Build history of the part. All positions in model axes, mm. Face numbers are marked on the shaded views. A direction names the side the tool comes from. Coordinates: 2 decimals unless noted, no trailing zeros. Order: outer loops, then holes, each group sorted by start corner. A loop starts at its lowest first (then second) coordinate and runs counter-clockwise, first axis right, second up. Notation, with made-up numbers: (-6.5, -34.75) - (1.5, -34.75) arc R18 ccw to (1.5, -12.75) - close; hole circle Ø1 at (-28, 41). An arc over 180 degrees is marked (long way). Return JSON: item names as keys, results as strings.
Autodesk Inventor part; units mm, degrees
ref_plane "YZ Plane" through (0, 0, 0) normal (1, 0, 0) x (0, 1, 0)
ref_plane "XZ Plane" through (0, 0, 0) normal (0, 1, 0) x (-1, 0, 0)
ref_plane "XY Plane" through (0, 0, 0) normal (0, 0, 1) x (1, 0, 0)
sketch "Skizze1" plane through (0, 0, 0) normal (0, 0, 1) x (1, 0, 0)
  line L0 (0, 0) -> (25, 0)
  line L1 (25, 0) -> (25, 30)
  line L2 (25, 30) -> (0, 30)
  line L3 (0, 30) -> (0, 0)
  dimension "d0" = 30
  dimension "d1" = 25
extrude "Extrusion1" add sketch "Skizze1" against normal blind 6
sketch "Skizze2" plane through (0, 0, 0) normal (0, 0, 1) x (1, 0, 0)
  circle A0 centre (12.5, 18) radius 8
  line L0 (25, 0) -> (25, 30)
  line L1 (0, 0) -> (25, 0)
  dimension "d4" = 16
  dimension "d5" = 12.5
  dimension "d6" = 18
extrude "Extrusion2" cut sketch "Skizze2" against normal blind 10
sketch "Skizze4" plane through (0, 0, 0) normal (0, 0, 1) x (1, 0, 0)
  line L0 (2.5, 13.3758) -> (22.5, 13.3758) construction
  line L1 (22.5, 13.3758) -> (22.5, 26.3758) construction
  line L2 (22.5, 26.3758) -> (2.5, 26.3758) construction
  line L3 (2.5, 26.3758) -> (2.5, 13.3758) construction
  line L4 (25, 0) -> (25, 30) construction
  circle A0 centre (2.5, 26.3758) radius 1.7
  circle A1 centre (22.5, 26.3758) radius 1.7
  circle A2 centre (22.5, 13.3758) radius 1.7
  circle A3 centre (2.5, 13.3758) radius 1.7
  point P0 (0, 0)
  point P1 (25, 3.0001)
  dimension "d12" = 20
  dimension "d13" = 13
  dimension "d14" = 2.5
  dimension "d15" = 3.4
  dimension "d16" = 3.4
  dimension "d17" = 3.4
  dimension "d18" = 3.4
extrude "Extrusion4" cut sketch "Skizze4" against normal blind 10
sketch "Skizze6" plane through (0, 0, 0) normal (0, 0, 1) x (1, 0, 0)
  line L0 (25, 0) -> (0, 0)
  line L1 (25, 0) -> (16, 0)
  line L2 (16, 0) -> (16, 6)
  line L3 (16, 6) -> (25, 6)
  line L4 (25, 6) -> (25, 0)
  line L5 (0, 0) -> (9, 0)
  line L6 (9, 0) -> (9, 6)
  line L7 (9, 6) -> (0, 6)
  line L8 (0, 6) -> (0, 0)
  line L9 (9, 6) -> (16, 6)
  line L10 (16, 6) -> (16, 0)
  line L11 (16, 0) -> (9, 0)
  line L12 (9, 0) -> (9, 6)
  dimension "d21" = 9
  dimension "d22" = 9
  dimension "d23" = 6
extrude "Extrusion5" cut sketch "Skizze6" against normal blind 10 contours L0 L6 L9 L2
sketch "Skizze7" plane through (0, 0, 0) normal (-1, 0, 0) x (0, 0, 1)
  circle A0 centre (-3, 2.5) radius 1.7
  line L0 (0, 30) -> (0, 0)
  line L1 (0, 0) -> (-6, 0)
  dimension "d26" = 3.4
  dimension "d27" = 3
  dimension "d28" = 2.5
extrude "Extrusion6" cut sketch "Skizze7" against normal blind 40
sketch "Skizze8" plane through (0, 0, 0) normal (0, 0, 1) x (1, 0, 0)
  line L0 (16, 6) -> (16, 0)
  line L1 (16, 0) -> (25, 0)
  line L2 (25, 0) -> (25, 30)
  line L3 (25, 30) -> (0, 30)
  line L4 (0, 30) -> (0, 0)
  line L5 (0, 0) -> (9, 0)
  line L6 (9, 0) -> (9, 6)
  line L7 (9, 6) -> (16, 6)
  circle A0 centre (22.5, 13.3758) radius 1.7
  circle A1 centre (2.5, 26.3758) radius 1.7
  circle A2 centre (22.5, 26.3758) radius 1.7
  circle A3 centre (2.5, 13.3758) radius 1.7
  circle A4 centre (12.5, 18) radius 8
  line L8 (0, 30) -> (0, 0)
  line L9 (0, 6) -> (25, 6)
  line L10 (25, 0) -> (25, 30)
  line L11 (25, 6) -> (25, 30)
  line L12 (25, 30) -> (0, 30)
  line L13 (25, 30) -> (0, 30)
  line L14 (0, 30) -> (0, 6)
extrude "Extrusion7" cut sketch "Skizze8" against normal blind 2 contours L7 L9 L4 L3 L2
properties part number "kamera ot" material "CFK"
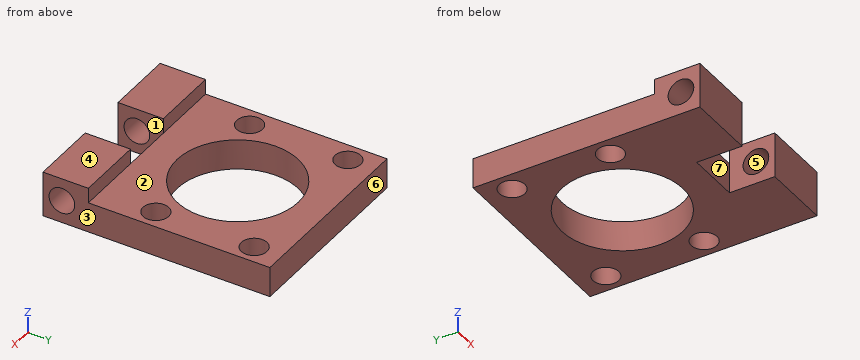
1. Mould opens along Y. For the marked faces 4, 5, 6 and 7 say: pulls with the +Y half, pulls with the -Y half, needs draft (parallel to the pull), parting line crosses it, or undercut.
Check values:
{"face 4": "needs draft", "face 5": "undercut", "face 6": "pulls with the +Y half", "face 7": "pulls with the -Y half"}
2. Probe L1, parallel to Y at x = 2.5, z = -3.15; L2, parallel to Y at x = 22.75, z = -4.1; L3, parallel to Y at x = 7, z = -0.8. List the from-to ranges inside material, lowest first.
Check values:
{"L1": "0 to 0.81, 4.19 to 11.68, 15.08 to 24.68, 28.08 to 30", "L2": "0 to 1.2, 3.8 to 11.69, 15.06 to 24.69, 28.06 to 30", "L3": "0 to 6"}
3. Cut at A-A on x = 2.5. Give the cut face in (y, z), plus the area to 3 significant figures.
Check values:
{"outline": "(0, -6) - (11.68, -6) - (11.68, -2) - (6, -2) - (6, 0) - (0, 0) - close; (15.08, -6) - (24.68, -6) - (24.68, -2) - (15.08, -2) - close; (28.08, -6) - (30, -6) - (30, -2) - (28.08, -2) - close; hole circle Ø3.4 at (2.5, -3)", "area": "95.7 mm²"}
4. Cut at D-D on y = 2.5. Give the cut face in (x, z), plus the area to 3 significant figures.
Check values:
{"outline": "(0, -6) - (9, -6) - (9, -4.7) - (0, -4.7) - close; (0, -1.3) - (9, -1.3) - (9, 0) - (0, 0) - close; (16, -6) - (25, -6) - (25, -4.7) - (16, -4.7) - close; (16, -1.3) - (25, -1.3) - (25, 0) - (16, 0) - close", "area": "46.8 mm²"}
5. Cut at C-C on z = -0.35. Give the cut face in (x, y).
Check values:
{"outline": "(0, 0) - (9, 0) - (9, 6) - (0, 6) - close; (16, 0) - (25, 0) - (25, 6) - (16, 6) - close"}
6. Tool access for the marked faces 1, 2 and 3: list every direction of +Z, -Z, +X, -X, +Y, -Y with a clear straight run to the whole face (end or side of a thin tool).
Check values:
{"face 1": "+Z, -Z, -Y", "face 2": "+Z, +X, -X, +Y", "face 3": "+Z, -Z, +X, +Y, -Y"}
7. Drop flat-ended pins along their axis: pin 1 (0.6 mm diameter, centred on x = 22.5, z = -1, fed in from +Y); pin 2 (14.5 mm diameter, centred on x = 12.5, y = 18, fed in from -Z); pin 3 (1.2 mm diameter, centred on x = 11, z = -4.5, fed in from -Y); pin 4 (4.5 mm diameter, centred on x = 2.5, y = 26.38, fed in from +Z). Give the stop position or say it passes through.
Check values:
{"pin 1": "y = 6", "pin 2": "through", "pin 3": "y = 6", "pin 4": "z = -2"}
8. Cut at B-B on y = 18. Give the cut face in (x, z), plus the area to 3 significant figures.
Check values:
{"outline": "(0, -6) - (4.5, -6) - (4.5, -2) - (0, -2) - close; (20.5, -6) - (25, -6) - (25, -2) - (20.5, -2) - close", "area": "36.0 mm²"}
